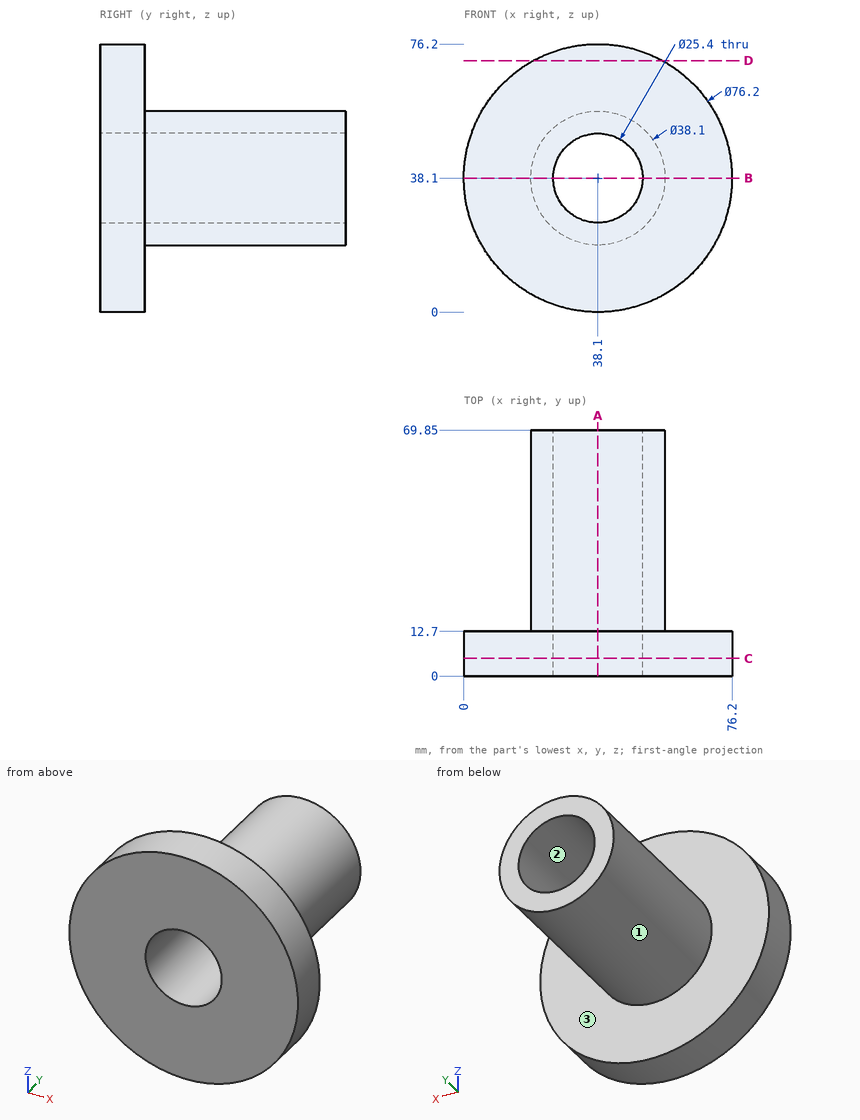
Can you work these out from the drawing? Everything is in mm from the part's minimum corner. Give positions to 0.01 mm unless a question says otherwise; leave off trailing zeros. Order: outer loops, then holes, each group sorted by start corner. A loop starts at its lowest first (then second) coordinate and runs counter-clockwise, first axis right, second up. Notation, with made-up numbers: M 41.5,82.25 L 71.5,82.25 A29 cw 71.5,105.25 Z; hole C 6.5,-30 d5. An arc over 180 degrees is marked long. Use a Markdown table: item, result. Add a question column.
1. For pin 1 Ø1.5 at (y, z) = (21, 28.5) entering from +X; pin 2 Ø4 at (x, y) = (57.5, 54.5) entering from +Z; pin 3 Ø1.5 at (x, y) = (26, 13.5) entering from -Z, each with a flat end and sliding along its axis, tell me the tip position at first contact or that it passes through.
2. Suppose I cut it at D-D (z = 71.5). List the corners of the cut face in (x, y) for me, and give its area (3 significant figures).
3. Suppose I cut it at B-B (z = 38.1). List the corners of the cut face in (x, y) for me.
4. Suppose I cut it at A-A (x = 38.1). List the corners of the cut face in (y, z) for me, and give its area (3 significant figures).
5. I need wall thicknesses on probe 1 along X at (y, z) = (18, 38.1); probe 2 along Y at (x, z) = (36, 4). Which ranges of each line are inside material? Lowest first, please. Write a range as from..to.
6. If we mould it in two halves opening along Z, with no side actions, what happens to the marked faces 1, 2 and 3? For each: +Z half, -Z half, draft (parallel to the pull), parting line (faces both ways), or undercut.
7. Suppose I cut it at C-C (y = 5). List the corners of the cut face in (x, z) for me, and give its area (3 significant figures).
Results list:
| question | item | result |
|---|---|---|
| 1 | pin 1 | stops at x = 54.97 |
| 1 | pin 2 | stops at z = 45.86 |
| 1 | pin 3 | stops at z = 22.8 |
| 2 | outline | M 19.77,0 L 56.43,0 L 56.43,12.7 L 19.77,12.7 Z |
| 2 | area | 466 mm² |
| 3 | outline | M 0,0 L 25.4,0 L 25.4,69.85 L 19.05,69.85 L 19.05,12.7 L 0,12.7 Z; M 50.8,0 L 76.2,0 L 76.2,12.7 L 57.15,12.7 L 57.15,69.85 L 50.8,69.85 Z |
| 4 | outline | M 0,0 L 12.7,0 L 12.7,19.05 L 69.85,19.05 L 69.85,25.4 L 0,25.4 Z; M 0,50.8 L 69.85,50.8 L 69.85,57.15 L 12.7,57.15 L 12.7,76.2 L 0,76.2 Z |
| 4 | area | 1,370 mm² |
| 5 | probe 1 | x = 19.05..25.4, 50.8..57.15 |
| 5 | probe 2 | y = 0..12.7 |
| 6 | face 1 | parting line |
| 6 | face 2 | undercut |
| 6 | face 3 | draft |
| 7 | outline | C 38.1,38.1 d76.2; hole C 38.1,38.1 d25.4 |
| 7 | area | 4,050 mm² |
